Autodesk Inventor part; units mm, degrees
ref_plane "YZ Plane" through (0, 0, 0) normal (1, 0, 0) x (0, 1, 0)
ref_plane "XZ Plane" through (0, 0, 0) normal (0, 1, 0) x (-1, 0, 0)
ref_plane "XY Plane" through (0, 0, 0) normal (0, 0, 1) x (1, 0, 0)
sketch "Sketch1" plane through (0, 0, 0) normal (0, 0, 1) x (1, 0, 0)
  circle A0 centre (0, 0) radius 1.25
  line L0 (0, -7) -> (0, 7)
  line L1 (-7.0223, 0) -> (7.1337, 0)
  line L2 (5, 5) -> (1.5, 5)
  line L3 (1.5, 5) -> (1.5, 4)
  line L4 (5, 5) -> (5, 1.5)
  line L5 (-1, 2) -> (1, 2)
  line L6 (2, 1) -> (2, -1)
  line L7 (1, -2) -> (-1, -2)
  line L8 (-2, -1) -> (-2, 1)
  line L9 (1, 2) -> (3.3835, 4)
  line L10 (2, 2) -> (4.1114, 2) construction
  line L11 (3.3835, 4) -> (1.5, 4)
  line L12 (2, 1) -> (4, 3.3835)
  line L13 (2, 1) -> (5.1114, 1) construction
  line L14 (5, 1.5) -> (4, 1.5)
  line L15 (4, 1.5) -> (4, 3.3835)
  line L16 (5, 5) -> (5, 1.5)
  line L17 (-5, 5) -> (-1.5, 5)
  line L18 (1.5, 5) -> (5, 5)
  line L19 (5, 5) -> (5, 1.5)
  line L20 (5, 0) -> (5, -5)
  line L21 (-2, 1) -> (-4, 3.3835)
  line L22 (-4, 3.3835) -> (-4, 1.5)
  line L23 (-5, 1.5) -> (-4, 1.5)
  line L24 (-5, 5) -> (-5, 1.5)
  line L25 (-5, 5) -> (-1.5, 5)
  line L26 (-1.5, 5) -> (-1.5, 4)
  line L27 (-1.5, 4) -> (-3.3835, 4)
  line L28 (-1, 2) -> (-3.3835, 4)
  line L29 (-1, -2) -> (-3.3835, -4)
  line L30 (-3.3835, -4) -> (-1.5, -4)
  line L31 (-1.5, -5) -> (-1.5, -4)
  line L32 (-5, -5) -> (-1.5, -5)
  line L33 (-5, -5) -> (-5, -1.5)
  line L34 (-5, -1.5) -> (-4, -1.5)
  line L35 (-4, -1.5) -> (-4, -3.3835)
  line L36 (-2, -1) -> (-4, -3.3835)
  line L37 (2, -1) -> (4, -3.3835)
  line L38 (4, -3.3835) -> (4, -1.5)
  line L39 (5, -1.5) -> (4, -1.5)
  line L40 (5, -5) -> (5, -1.5)
  line L41 (5, -5) -> (1.5, -5)
  line L42 (1.5, -5) -> (1.5, -4)
  line L43 (1.5, -4) -> (3.3835, -4)
  line L44 (1, -2) -> (3.3835, -4)
  line L45 (-5, -5) -> (-5, -1.5)
  line L46 (-5, 1.5) -> (-5, 5)
  line L47 (5, -5) -> (1.5, -5)
  line L48 (-1.5, -5) -> (-5, -5)
  dimension "d0" = 2.5
  dimension "d3" = 3.5
  dimension "d4" = 1
  dimension "d5" = 90
  dimension "d6" = 3.5
  dimension "d10" = 2
  dimension "d11" = 40
  dimension "d13" = 50
  dimension "d14" = 1
  dimension "d17" = 360
  dimension "d19" = 3.1115
extrude "Extrusion1" add sketch "Sketch1" along normal mid plane 100 contours L1 L6 L37 L38 L39 L20 L41 L42 L43 L44 L7 L0 A0 | A0 L0 L5 L9 L11 L3 L2 L4 L14 L15 L12 L6 L1 | A0 L1 L8 L21 L22 L23 L24 L17 L26 L27 L28 L5 L0 | L0 L7 L29 L30 L31 L32 L33 L34 L35 L36 L8 L1 A0
fillet "Fillet1" radius 0.18 28 edges at (-5, 5, 0) (-5, 1.5, 0) (-1.5, 5, 0) (-1.5, 4, 0) (-4, 1.5, 0) (-3.3835, 4, 0) (-4, 3.3835, 0) (1.5, 5, 0) (5, 5, 0) (3.3835, 4, 0) (4, 3.3835, 0) (4, 1.5, 0) (5, 1.5, 0) (1.5, 4, 0) (4, -1.5, 0) (5, -1.5, 0) (5, -5, 0) (4, -3.3835, 0) (3.3835, -4, 0) (1.5, -4, 0) (1.5, -5, 0) (-3.3835, -4, 0) (-4, -3.3835, 0) (-4, -1.5, 0) (-5, -1.5, 0) (-5, -5, 0) (-1.5, -5, 0) (-1.5, -4, 0)
fillet "Fillet2" radius 0.3 8 edges at (-1, 2, 0) (1, 2, 0) (2, -1, 0) (2, 1, 0) (1, -2, 0) (-1, -2, 0) (-2, -1, 0) (-2, 1, 0)
thread "Thread1"
thread "Thread2"
properties part number "Beam_10mm"
The model under review builds one solid part; all positions refer to its coordinate system, in mm. A direction names the side the tool comes from. Round coordinates to 2 decimals unless told otherwise and drop trailing zeros. Order: outer loops, then holes, each group sorted by start corner. A loop starts at its lowest first (then second) coordinate and runs counter-clockwise, first axis right, second up.
(1) For P1, Ø3, axis at x = 0, y = 0, coming from the -Z side; P2, Ø0.5, axis at y = 0, z = 0, coming from the +X side, all flat-tipped, find the tip position at first contact; note any pin that passes through.
Working result:
P1: stops at z = -50
P2: stops at x = 2
(2) Take a section at A-A, the plane y = 0. State the section outline as (x, z) points.
Working result:
outline: (-2, -50) - (-1.25, -50) - (-1.25, 50) - (-2, 50) - close; (1.25, -50) - (2, -50) - (2, 50) - (1.25, 50) - close
(3) Wall thickness on L1, parallel to Y at x = -3.75, z = -9.5; L2, parallel to X at y = -4.25, z = 3; L3, parallel to X at y = 0, z = -21.5: over which ranges is each line inside the solid? List them lowest first.
Working result:
L1: y = -5 to -3.05, 3.05 to 5
L2: x = -5 to -1.5, 1.5 to 5
L3: x = -2 to -1.25, 1.25 to 2
(4) Mouldability with a two-part tool opening along Y and no side actions: class faces 4 (the face through (-5, 3, -1)), 5 (the face through (-3, 5, -1)), 6 (the face through (-0.27, 1.22, -0.7)) as released by +Y, released by -Y, zero draft, split by the parting line, or undercut.
Working result:
face 4: zero draft
face 5: released by +Y
face 6: undercut
(5) Tool access review of faces 1 (the face through (-2.865, 2.031, -0.7)), 2 (the face through (2, 0, -1)), 3 (the face through (-2, 0, -1)): name each direction out of +Z, -Z, +X, -X, +Y, -Y from which nothing blocks a thin tool from reaching the whole face with its end or side.
Working result:
face 1: +Z, -Z
face 2: +Z, -Z, +X
face 3: +Z, -Z, -X
